Can you work these out from the model? Positions are in its coordinate system, mm. A direction names the side the tool comes from. Give positions to 0.01 mm unless a question says otherwise; leave off trailing zeros. Order: outer loops, then holes, each group sorted by start corner. A loop starts at its lowest first (then second) coordinate and runs counter-clockwise, first axis right, second up. Notation, with made-up numbers: M 71,74.25 L 94,74.25 A38 cw 94,113.25 Z; hole C 2.5,81 d3. An arc over 180 degrees is marked long. Use a Markdown table: item, result. Add a question column.
from build123d import *

# Parameters (mm, degrees)
F0_R      = 25
F1_DEPTH  = 5
F2_R      = 2.65
F3_DEPTH  = 5
F5_R      = 18.238073
F6_DEPTH  = 10
F7_R      = 14.619557
F8_DEPTH  = 10
F9_R      = 2.787227
F10_DEPTH = 10
F12_DEPTH = 2
F13_R     = 1.869592
F14_DEPTH = 25.4


with BuildPart() as f1:
    # F0 (on Front) → F1 (new body)
    with BuildSketch(Plane.XZ):
        Circle(F0_R)
    extrude(amount=F1_DEPTH)

    # F2 (on face) → F3 (cut)
    with BuildSketch(Plane(origin=(0, 0, 0), x_dir=(-1, 0, 0), z_dir=(0, 1, 0))):
        Circle(F2_R)
    extrude(amount=-F3_DEPTH, mode=Mode.SUBTRACT)

    # F5 (on face) → F6 (join)
    with BuildSketch(Plane.XZ.offset(5)):
        with Locations((-0.701384, 0)):
            Circle(F5_R)
    extrude(amount=F6_DEPTH)

    # F7 (on face) → F8 (cut)
    with BuildSketch(Plane.XZ.offset(15)):
        Circle(F7_R)
    extrude(amount=-F8_DEPTH, mode=Mode.SUBTRACT)

    # F9 (on face) → F10 (join)
    with BuildSketch(Plane.XZ.offset(5)):
        with Locations((0, 21.991307)):
            Circle(F9_R)
    extrude(amount=F10_DEPTH)

    # F11 (on face) → F12 (join)
    with BuildSketch(Plane.XZ.offset(15)):
        with BuildLine():
            Line((-2.749703, 22.447126), (-3.600255, 22.447126))
            Line((-3.600255, 22.447126), (-3.600255, 14.876149))
            Line((-3.600255, 14.876149), (3.30658, 14.876149))
            Line((3.30658, 14.876149), (3.30658, 22.447126))
            Line((3.30658, 22.447126), (2.749703, 22.447126))
            ThreePointArc((2.749703, 22.447126), (2.77783, 22.219987), (2.787227, 21.991307))
            ThreePointArc((2.787227, 21.991307), (-0.228681, 19.213476), (-2.749703, 22.447126))
        make_face()
        with BuildLine():
            Line((2.749703, 22.447126), (-2.749703, 22.447126))
            ThreePointArc((-2.749703, 22.447126), (-0.228681, 19.213476), (2.787227, 21.991307))
            ThreePointArc((2.787227, 21.991307), (2.77783, 22.219987), (2.749703, 22.447126))
        make_face()
    extrude(amount=F12_DEPTH)

    # F13 (on face) → F14 (cut)
    with BuildSketch(Plane.YZ.offset(3.30658)):
        with Locations((-10.008663, 22.004483)):
            Circle(F13_R)
    extrude(amount=-F14_DEPTH, mode=Mode.SUBTRACT)


solid = f1.part
1. If we section it at D-D, the plane z = 17: List the corners of the cut face in (x, y) for me.
2. Will these pins go through, and if not, where does the flat tip stop? pin 1 (6 mm diameter, centred on y = -6.5, z = -8.5, fed in from -X); pin 2 (1.2 mm diameter, centred on x = -0.5, z = 24, fed in from -Y); pin 3 (0.6 mm diameter, centred on y = -15.5, z = 20, fed in from -X).
3. If we section it at C-C, the plane y = -8.75: List the corners of the cut face in (x, z) for me.
4. If we section it at A-A, the plane z = 0: List the corners of the cut face in (x, y) for me, then the cut area to 3 significant figures.
5. On a 3-axis mill with a long thin cutter (end or side, diameter ignored), from which of +Z, -Z, +X, -X, +Y, -Y can I reach the whole of each face in a straight line? I mean faces 4 (the face through (-3.6, -16, 19)), 5 (the face through (0, -15, 19)), 6 (the face through (0, -15, 23)), 7 (the face through (0, -5, -3)), 8 (the face through (3.307, -16, 19)). Say none if no direction works.
6. I need wall thicknesses on L1, parallel to Z at x = 0, y = -12; L2, parallel to Z at x = 0, y = -11; L3, parallel to Z at x = 0, y = -2.65. Which ranges of each line are inside material? Lowest first, please. Write a range as [from, to].
7. If we section it at B-B, the plane x = 1: List the corners of the cut face in (y, z) for me.
8. We'd pull the mould along Z, two halves only. Please class faces 1 (the face through (0, -16, 22.447)), 2 (the face through (6.75, -10.07, -12.97)), 3 (the face through (0, -16, 14.876)): +Z half, -Z half, draft (parallel to the pull), parting line (faces both ways), or undercut.
Geometry results:
| question | item | result |
|---|---|---|
| 1 | outline | M -18.33,-5 L -7.31,-5 L -7.31,-15 L -3.6,-15 L -3.6,-17 L 3.31,-17 L 3.31,-15 L 5.9,-15 L 5.9,-5 L 18.33,-5 L 18.33,0 L -18.33,0 Z |
| 2 | pin 1 | stops at x = -24.29 |
| 2 | pin 2 | stops at y = -15 |
| 2 | pin 3 | stops at x = -3.6 |
| 3 | outline | C -0.7,0 d36.48; M -2.43,20.62 A2.79 ccw 2.43,20.62 Z; M -2.41,23.39 L 2.41,23.39 A2.79 ccw Z; hole C 0,0 d29.24 |
| 4 | outline | M -25,-5 L -18.94,-5 L -18.94,-15 L -14.62,-15 L -14.62,-5 L -2.65,-5 L -2.65,0 L -25,0 Z; M 2.65,-5 L 14.62,-5 L 14.62,-15 L 17.54,-15 L 17.54,-5 L 25,-5 L 25,0 L 2.65,0 Z |
| 4 | area | 296 mm^2 |
| 5 | face 4 | +Z, -Z, -X, -Y |
| 5 | face 5 | none |
| 5 | face 6 | +Z, +X, -X, -Y |
| 5 | face 7 | -Y |
| 5 | face 8 | +Z, -Z, +X, -Y |
| 6 | L1 | z = [-18.22, -14.62], [14.62, 18.22], [19.2, 24.78] |
| 6 | L2 | z = [-18.22, -14.62], [14.62, 18.22], [19.2, 20.42], [23.59, 24.78] |
| 6 | L3 | z = [-25, -2.65], [2.65, 25] |
| 7 | outline | M -17,14.88 L -15,14.88 L -15,14.59 L -5,14.59 L -5,2.45 L 0,2.45 L 0,24.98 L -5,24.98 L -5,24.59 L -15,24.59 L -15,22.45 L -17,22.45 Z; M -15,-18.16 L -5,-18.16 L -5,-24.98 L 0,-24.98 L 0,-2.45 L -5,-2.45 L -5,-14.59 L -15,-14.59 Z; hole M -15,18.16 L -5,18.16 L -5,19.39 L -15,19.39 Z; hole C -10.01,22 d3.74 |
| 8 | face 1 | +Z half |
| 8 | face 2 | undercut |
| 8 | face 3 | -Z half |
